Source: CAD feature listing. Evaluate the final solid. Frame: model axes, mm. Face numbers are marked on the shaded views. Coordinates: 2 decimals unless noted, no trailing zeros. Order: outer loops, then holes, each group sorted by start corner. A loop starts at its lowest first (then second) coordinate and runs counter-clockwise, first axis right, second up.
```python
from build123d import *

# Parameters (mm, degrees)
ESQUISSE1_R        = 2
ESQUISSE1_R_2      = 2.146897886
BOSS_EXTRU_1_DEPTH = 1


with BuildPart() as part:
    # Esquisse1 → Boss.-Extru.1 (new body)
    with BuildSketch(Plane.XY):
        with BuildLine():
            Line((-95, -31.75), (95, -31.75))
            ThreePointArc((95, -31.75), (107.515790027, -26.565790027), (112.7, -14.05))
            Line((112.7, -14.05), (112.7, 14.05))
            ThreePointArc((112.7, 14.05), (107.515790027, 26.565790027), (95, 31.75))
            Line((95, 31.75), (-95, 31.75))
            ThreePointArc((-95, 31.75), (-107.515790027, 26.565790027), (-112.7, 14.05))
            Line((-112.7, 14.05), (-112.7, -14.05))
            ThreePointArc((-112.7, -14.05), (-107.515790027, -26.565790027), (-95, -31.75))
        make_face()
        with Locations((-106.2, 0)):
            Circle(ESQUISSE1_R, mode=Mode.SUBTRACT)
        with Locations((0, 25.25)):
            Circle(ESQUISSE1_R, mode=Mode.SUBTRACT)
        with Locations((-95, 25.25)):
            Circle(ESQUISSE1_R_2, mode=Mode.SUBTRACT)
        with Locations(Location((-95, -25.25, 0), (0, 0, 180))):
            Circle(ESQUISSE1_R_2, mode=Mode.SUBTRACT)
        with Locations(Location((0, -25.25, 0), (0, 0, 180))):
            Circle(ESQUISSE1_R, mode=Mode.SUBTRACT)
        with Locations((95, -25.25)):
            Circle(ESQUISSE1_R_2, mode=Mode.SUBTRACT)
        with Locations(Location((106.2, 0, 0), (0, 0, 180))):
            Circle(ESQUISSE1_R, mode=Mode.SUBTRACT)
        with Locations(Location((95, 25.25, 0), (0, 0, 180))):
            Circle(ESQUISSE1_R_2, mode=Mode.SUBTRACT)
        with BuildLine():
            Line((-95, -19.05), (95, -19.05))
            ThreePointArc((95, -19.05), (98.535533906, -17.585533906), (100, -14.05))
            Line((100, -14.05), (100, 14.05))
            ThreePointArc((100, 14.05), (98.535533906, 17.585533906), (95, 19.05))
            Line((95, 19.05), (-95, 19.05))
            ThreePointArc((-95, 19.05), (-98.535533906, 17.585533906), (-100, 14.05))
            Line((-100, 14.05), (-100, -14.05))
            ThreePointArc((-100, -14.05), (-98.535533906, -17.585533906), (-95, -19.05))
        make_face(mode=Mode.SUBTRACT)
    extrude(amount=BOSS_EXTRU_1_DEPTH)


solid = part.part
```
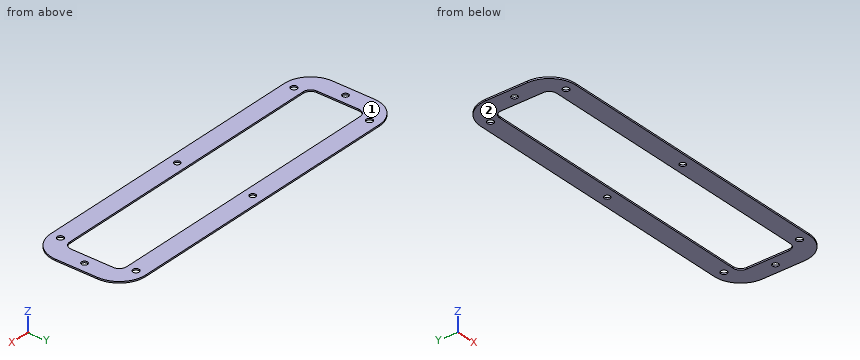
Q1. Section query A-A on y = 0. Output: boundary loops of the cut face in (x, z).
Solutions:
outline: (-112.7, 0) - (-108.2, 0) - (-108.2, 1) - (-112.7, 1) - close; (-104.2, 0) - (-100, 0) - (-100, 1) - (-104.2, 1) - close; (100, 0) - (104.2, 0) - (104.2, 1) - (100, 1) - close; (108.2, 0) - (112.7, 0) - (112.7, 1) - (108.2, 1) - close
Q2. Section query D-D on x = -30.5. Output: boundary loops of the cut face in (y, z).
Solutions:
outline: (-31.75, 0) - (-19.05, 0) - (-19.05, 1) - (-31.75, 1) - close; (19.05, 0) - (31.75, 0) - (31.75, 1) - (19.05, 1) - close
Q3. Section query C-C on z = 0.55. Give the number of separate pieces and of enclosed holes in the cut face, plus the area to 3 significant figures.
Solutions:
separate pieces: 1
enclosed holes: 9
area: 6,340 mm2
Q4. Section query B-B on x = 0. Output: boundary loops of the cut face in (y, z), plus the area to 3 significant figures.
Solutions:
outline: (-31.75, 0) - (-27.25, 0) - (-27.25, 1) - (-31.75, 1) - close; (-23.25, 0) - (-19.05, 0) - (-19.05, 1) - (-23.25, 1) - close; (19.05, 0) - (23.25, 0) - (23.25, 1) - (19.05, 1) - close; (27.25, 0) - (31.75, 0) - (31.75, 1) - (27.25, 1) - close
area: 17.4 mm2
Q5. Pin query (flat end, axial travel): P1, Ø3.5, axis at x = 95, y = 25.25, coming from the -Z side. Return the tip coordinate at first contact, or that it passes through.
Solutions:
P1: passes through
Q6. Material intervals for line 1 along Y through (x, z) = (95, 0.2); line 2 along Y through (x, z) = (0, 0.6); line 3 along X through (y, z) = (-13, 0.75), sorted ascending.
Solutions:
line 1: y = -31.75 to -27.4, -23.1 to -19.05, 19.05 to 23.1, 27.4 to 31.75
line 2: y = -31.75 to -27.25, -23.25 to -19.05, 19.05 to 23.25, 27.25 to 31.75
line 3: x = -112.7 to -100, 100 to 112.7
Q7. Pull-direction query (Z, two-part tool) for the marked faces 1 and 2; classes: pulls with the +Z half, pulls with the -Z half, needs draft (parallel to the pull), parting line crosses it, or undercut.
Solutions:
face 1: pulls with the +Z half
face 2: pulls with the -Z half
